The model under review builds one solid part; all positions refer to its coordinate system, in mm. A direction names the side the tool comes from. Round coordinates to 2 decimals unless told otherwise and drop trailing zeros. Order: outer loops, then holes, each group sorted by start corner. A loop starts at its lowest first (then second) coordinate and runs counter-clockwise, first axis right, second up. Notation, with made-up numbers: M 70,20 L 117,20 A21 ccw 117,58 Z; hole C 68.5,7.25 d9. An arc over 180 degrees is marked long. Answer as a JSON object with one key per item and string values. Group by question number.
1. Add section A-A on y = -19.5. State the section outline as (x, z) points.
2. Add section C-C on y = 6. State the section outline as (x, z) points.
3. To check wall thickness, follow probe 1 along X at (y, z) = (4.5, 1.6); probe 2 along Y at (x, z) = (5.5, 1.2); probe 3 along Y at (x, z) = (-20, 0.4). State the ranges of each line that lie inside material, in increasing order. Write a range as [from, to].
4. Mouldability with a two-part tool opening along Y and no side actions: class faces 4 (the face through (9.237, 22.767, 4.532)), 5 (the face through (2, 28, 2)), 6 (the face through (0, 14, 2)), 7 (the face through (-3, -7, 0)) as released by +Y, released by -Y, zero draft, split by the parting line, or undercut.
5. Machinability: for faces 1 (the face through (-37.5, -8, 4.5)), 2 (the face through (0, -9, 2)), 3 (the face through (-37.5, -8, 0.5)), which of the approach directions +Z, -Z, +X, -X, +Y, -Y give a long, thin tool a straight path to every point of the face, cutting with its end or side? Answer none if there is none.
6. Add section B-B on x = -20. State the section outline as (y, z) points.
7. Clearance check with flat-ended pins moving along their axes: P1, Ø1.5, axis at x = -35, z = 2.5, coming from the -Y side; P2, Ø2, axis at x = -27.5, z = 2, coming from the -Y side; P3, Ø1.5, axis at y = 19.5, z = 3, coming from the +X side. State where each tip first meets the part, or that it passes through.
```python
from build123d import *

# Parameters (mm, degrees)
EXTRUDE_1_DEPTH     = 5
FILLET_1_R          = 2.5
FILLET_2_R          = 1
EXTRUDE_2_DEPTH     = 8
FILLET_3_R          = 2.5
SKETCH_5_W          = 1.467751534
SKETCH_5_H          = 4.178210798
SKETCH_5_W_2        = 1.389566385
CUT_EXTRUDE_1_DEPTH = 20


with BuildPart() as part:
    # 草图1 → 凸台-拉伸1 (new body)
    with BuildSketch(Plane.XY):
        with BuildLine():
            Line((0, 0), (0, 28))
            Line((0, 28), (4, 28))
            Line((4, 28), (7.380946094, 20.749537704))
            Line((7.380946094, 20.749537704), (11.912485029, 22.862629012))
            Line((11.912485029, 22.862629012), (7.185351304, 33))
            Line((7.185351304, 33), (-5, 33))
            Line((-5, 33), (-5, -12))
            ThreePointArc((-5, -12), (-20, -27), (-35, -12))
            Line((-35, -12), (-35, -7))
            Line((-35, -7), (-40, -7))
            Line((-40, -7), (-40, -12))
            ThreePointArc((-40, -12), (-20, -32), (0, -12))
            Line((0, -12), (0, -5))
            Line((0, -5), (8, -5))
            Line((8, -5), (8, 0))
            Line((8, 0), (0, 0))
        make_face()
    extrude(amount=EXTRUDE_1_DEPTH)

    # 圆角1
    fillet_1_edges = [part.edges().sort_by_distance(p)[0] for p in [
        (-37.5, -7, 0),
        (9.646715562, 21.806083358, 0),
        (9.646715562, 21.806083358, 5),
        (-40, -7, 2.5),
        (-35, -7, 2.5),
        (7.185351304, 33, 2.5),
        (11.912485029, 22.862629012, 2.5),
        (7.380946094, 20.749537704, 2.5),
        (-37.5, -7, 5),
    ]]
    fillet(fillet_1_edges, radius=FILLET_1_R - 0.0001)  # a hair under: the kernel refuses the full size

    # 圆角2
    fillet_2_edges = [part.edges().sort_by_distance(p)[0] for p in [
        (-5, 33, 2.5),
    ]]
    fillet(fillet_2_edges, radius=FILLET_2_R)

    # 草图3 → 凸台-拉伸2 (add)
    with BuildSketch(Plane(origin=(0, 0, 0), x_dir=(0, 0, -1), z_dir=(1, 0, 0))):
        with BuildLine():
            Line((-5, 0), (0, 0))
            ThreePointArc((0, 0), (-2.5, 2.5), (-5, 0))
        make_face()
    extrude(amount=EXTRUDE_2_DEPTH)

    # 圆角3
    fillet_3_edges = [part.edges().sort_by_distance(p)[0] for p in [
        (8, -2.5, 0),
        (8, -5, 2.5),
        (8, -2.5, 5),
        (8, 2.5, 2.5),
    ]]
    fillet(fillet_3_edges, radius=FILLET_3_R - 0.0001)  # a hair under: the kernel refuses the full size

    # 草图4 → 旋转3 (revolve)
    with BuildSketch(Plane(origin=(4.4, 0, 0), x_dir=(0, 0, -1), z_dir=(1, 0, 0))):
        with BuildLine():
            Line((-5.5, 0), (0.5, 0))
            ThreePointArc((0.5, 0), (-2.5, 3), (-5.5, 0))
        make_face()
    revolve(axis=Axis((4.4, 0, 2.5), (0, 0, -1)))

    # 草图5 → 切除-拉伸1 (cut)
    with BuildSketch(Plane.ZY.offset(5)):
        with Locations((-0.733875767, -0.010051234)):
            Rectangle(SKETCH_5_W, SKETCH_5_H)
        with Locations((5.694783193, -0.010051234)):
            Rectangle(SKETCH_5_W_2, SKETCH_5_H)
    extrude(amount=-CUT_EXTRUDE_1_DEPTH, mode=Mode.SUBTRACT)


solid = part.part
```
Recorded:
{
 "1": {"outline": "M -38.54,0 L -32.99,0 L -32.99,5 L -38.54,5 Z; M -7.01,0 L -1.46,0 L -1.46,5 L -7.01,5 Z"},
 "2": {"outline": "M -5,0 L 0,0 L 0,5 L -5,5 Z"},
 "3": {"probe 1": "x = [-5, 0]", "probe 2": "y = [-5, 2.47], [24.78, 33]", "probe 3": "y = [-32, -27]"},
 "4": {"face 4": "released by -Y", "face 5": "undercut", "face 6": "undercut", "face 7": "zero draft"},
 "5": {"face 1": "+Z, -X, +Y", "face 2": "+Z, -Z, +X, -Y", "face 3": "-Z, -X, +Y"},
 "6": {"outline": "M -32,0 L -27,0 L -27,5 L -32,5 Z"},
 "7": {"P1": "stops at y = -26.03", "P2": "stops at y = -30.91", "P3": "stops at x = 0"}
}
